Solid Edge part; units mm, degrees
sketch "Sketch1" plane through (0, 0, 0) normal (0, 0, 1) x (1, 0, 0)
  line L0 (-37, -38.5) -> (37, -38.5)
  line L1 (37, -38.5) -> (37, 38.5)
  line L2 (37, 38.5) -> (-37, 38.5)
  line L3 (-37, 38.5) -> (-37, -38.5)
  dimension "D1" = 37
  dimension "D2" = 37
extrude "Ajout_matière_1" add sketch "Sketch1" along normal blind 36
sketch "Sketch2" plane through (0, -38.5, 18) normal (0, -1, 0) x (1, 0, 0)
  circle A0 centre (23, 5) radius 4
extrude "Cutout1" cut sketch "Sketch2" along normal through all and the other way through all
sketch "Sketch3" plane through (0, 0, 0) normal (0, 0, 1) x (1, 0, 0)
  line L0 (37, 38.5) -> (66, 38.5)
  line L1 (66, 38.5) -> (66, 27.2)
  line L2 (66, 27.2) -> (37, 27.2)
  line L3 (37, 27.2) -> (37, 38.5)
  line L4 (37, -38.5) -> (66, -38.5)
  line L5 (66, -38.5) -> (66, -28.5)
  line L6 (66, -28.5) -> (37, -28.5)
  line L7 (37, -28.5) -> (37, -38.5)
  line L8 (37, 6.3) -> (66, 6.3)
  line L9 (66, 6.3) -> (66, -5)
  line L10 (66, -5) -> (37, -5)
  line L11 (37, -5) -> (37, 6.3)
  dimension "D1" = 66
  dimension "D2" = 37
  dimension "D3" = 66
  dimension "D4" = 66
  dimension "D5" = 66
  dimension "D6" = 66
extrude "Ajout_matière_2" add sketch "Sketch3" along normal blind 9
sketch "Sketch4" plane through (14.5, -38.5, 18) normal (0, -1, 0) x (1, 0, 0)
  line L0 (-51.5, -18) -> (0.5, -18)
  line L1 (0.5, -18) -> (0.5, 10.5)
  line L2 (0.5, 10.5) -> (-51.5, 10.5)
  line L3 (-51.5, 10.5) -> (-51.5, -18)
  dimension "D1" = 0.5
  dimension "D2" = 0.5
extrude "Cutout2" cut sketch "Sketch4" against normal through all
sketch "Sketch5" plane through (14.5, -38.5, 18) normal (0, -1, 0) x (1, 0, 0)
  line L0 (0.5, -18) -> (10.3402, -18)
  line L1 (10.3402, -18) -> (10.3402, 6.2121)
  line L2 (7.6235, 6.2121) -> (10.3402, 6.2121)
  line L3 (7.6235, 10.5) -> (7.6235, 6.2121)
  line L4 (0.5, 10.5) -> (7.6235, 10.5)
  line L5 (0.5, 10.5) -> (0.5, 6.2121)
  line L6 (0.5, 6.2121) -> (0.5, -18)
extrude "Cutout3" cut sketch "Sketch5" against normal through all
sketch "Sketch6" plane through (0, 0, 36) normal (0, 0, 1) x (1, 0, 0)
  line L0 (-34.62, -36.28) -> (34.62, -36.28)
  line L1 (34.62, -36.28) -> (34.62, 36.28)
  line L2 (34.62, 36.28) -> (-34.62, 36.28)
  line L3 (-34.62, 36.28) -> (-34.62, -36.28)
  dimension "D1" = 34.62
  dimension "D2" = 34.62
extrude "Enlèvement_matière_5" cut sketch "Sketch6" against normal blind 5
hole "Perçage_1" at (17.62, 7.28, 31) direction (0, 0, -1) diameter 4.5 end up to next
hole "Hole1" at (17.62, -7.28, 31) direction (0, 0, -1) diameter 4.5 end up to next
properties material "Nylon, usage général"
Can you work these out from the model? Positions are in its coordinate system, mm. A direction names the side the tool comes from. Coordinates: 2 decimals unless noted, no trailing zeros. Loops run counter-clockwise (first coordinate to the right, second up) from the corner with the lowest first, then second, coordinate; pieces in that order, holes last. Notation, with made-up numbers: M -28,-33 L -7,-33 A15 cw -7,-14 Z; hole C -24,62.5 d7. An arc over 180 degrees is marked long. Return JSON: item names as keys, results as strings. Group by question number.
Item 1: If I drill on L1, parallel to Y at x = 17.62, z = 30.45; L2, parallel to X at y = 7.28, z = 29.85; L3, parallel to Y at x = 17, z = 29, over which ranges is the centre line in solid material (lowest first)? Write a range as from..to.
Item 2: Imagine slicing it at C-C (x = -20). Please give me the cut outline in (y, z), and give its area (3 significant figures).
Item 3: Thinking about a two-plate mould opening in Z: for faces 5 (the flat face through (52, -5, 4)), 6 (the cylindrical face through (26.785, -0.539, 24.293)), 7 (the flat face through (-36, 0, 36)), which applies, released by +Z, released by -Z, zero draft, split by the parting line, or undercut?
Item 4: Imagine slicing it at B-B (x = 17.62). Please give me the cut outline in (y, z), and give its area (3 significant figures).
Item 5: Imagine slicing it at A-A (y = -7.28). Please give me the cut outline in (x, z), and give its area (3 significant figures).
Item 6: On a 3-axis mill with a long thin cutter (end or side, diameter ignored), from which of +Z, -Z, +X, -X, +Y, -Y can I reach the whole of each face in a straight line? I mean faces 1 (the flat face through (0, 36.28, 34)), 2 (the flat face through (52, 33, 9)), 3 (the flat face through (24.84, -1, 10)), 4 (the flat face through (52, 27.2, 4)). Say none if no direction works.
Item 7: Imagine slicing it at D-D (z = 14). Please give me the cut outline in (x, y).
Item 8: I'm going to push flat-ended pins straight in: pin 1 Ø3 at (x, y) = (26, -8.5) entering from +Z; pin 2 Ø8 at (x, y) = (40, -16.5) entering from -Z; pin 3 Ø1 at (y, z) = (-13.5, 4.5) entering from +X; pin 4 Ø3 at (y, z) = (-22.5, 20.5) entering from -X. Where does each tip first touch, or does it pass through?
Verdict:
{
 "1": {"L1": "y = -38.5..-9.53, -5.03..5.03, 9.53..38.5", "L2": "x = -37..15.37, 19.87..37", "L3": "y = -38.5..-9.44, -5.12..5.12, 9.44..38.5"},
 "2": {"outline": "M -38.5,28.5 L 38.5,28.5 L 38.5,36 L 36.28,36 L 36.28,31 L -36.28,31 L -36.28,36 L -38.5,36 Z", "area": "215 mm^2"},
 "3": {"face 5": "zero draft", "face 6": "undercut", "face 7": "released by +Z"},
 "4": {"outline": "M -38.5,28.5 L -9.53,28.5 L -9.53,31 L -36.28,31 L -36.28,36 L -38.5,36 Z; M -5.03,28.5 L 5.03,28.5 L 5.03,31 L -5.03,31 Z; M 9.53,28.5 L 38.5,28.5 L 38.5,36 L 36.28,36 L 36.28,31 L 9.53,31 Z", "area": "192 mm^2"},
 "5": {"outline": "M -37,28.5 L 15.37,28.5 L 15.37,31 L -34.62,31 L -34.62,36 L -37,36 Z; M 19.87,28.5 L 22.12,28.5 L 22.12,26.9 A4 cw 24.84,19.45 L 24.84,0 L 37,0 L 37,36 L 34.62,36 L 34.62,31 L 19.87,31 Z", "area": "538 mm^2"},
 "6": {"face 1": "+Z", "face 2": "+Z, +X, +Y, -Y", "face 3": "-Z, -X, +Y, -Y", "face 4": "+Z, -Z, +X"},
 "7": {"outline": "M 24.84,-38.5 L 37,-38.5 L 37,38.5 L 24.84,38.5 Z"},
 "8": {"pin 1": "stops at z = 31", "pin 2": "stops at z = 0", "pin 3": "stops at x = 37", "pin 4": "stops at x = 24.84"}
}
